Here's how the part is built. I have some questions about the finished solid (model axes, mm). Face numbers are marked on the shaded views. A direction names the side the tool comes from. Coordinates: 2 decimals unless noted, no trailing zeros. Loops run counter-clockwise (first coordinate to the right, second up) from the corner with the lowest first, then second, coordinate; pieces in that order, holes last. Notation, with made-up numbers: M -27.5,30.25 L -9.5,30.25 A24 cw -9.5,68.25 Z; hole C -6.5,38 d5. An arc over 180 degrees is marked long. Use one line per item in the form item = value. Start each with the question number.
(1) On a 3-axis mill with a long thin cutter (end or side, diameter ignored), from which of +Z, -Z, +X, -X, +Y, -Y can I reach the whole of each face in a straight line? I mean the marked faces 4, 5 and 6. Say none if no direction works.
(2) Imagine slicing it at C-C, the plane y = 38. Please give me the cut outline in (x, z), and give its area (3 significant figures).
(3) Thinking about a two-plate mould opening in Z: for the marked faces 1, 2 and 3, which applies, +Z half, -Z half, draft (parallel to the pull), parting line (faces both ways), or undercut?
(4) Imagine slicing it at B-B, the plane x = -43.5. Please give me the cut outline in (y, z).
(5) Imagine slicing it at D-D, the plane z = 31. Please give me the cut outline in (x, y).
(6) Please list where these lines run through material, in increasing order: L1, parallel to Z at x = 33, y = 51.5; L2, parallel to Z at x = 9, y = 14.5; L3, parallel to Y at x = -36.5, z = 63.5.
(7) Imagine slicing it at A-A, the plane y = 19. Please give me the cut outline in (x, z), and give its area (3 significant figures).
(8) Will these pins go through, and if not, where does the flat tip stop? P1, Ø4, axis at x = -13, z = 35.5, coming from the -Y side; P2, Ø9.5, axis at x = -26.5, z = 65.5, coming from the +Y side; P3, Ø1, axis at x = -31.5, y = 26.5, coming from the +Z side.
```python
from build123d import *

# Parameters (mm, degrees)
F0_W        = 100.3427430987
F0_H        = 68.4072636068
F1_DEPTH    = 75
F2_T1_DEPTH = 460.378361414
F3_W        = 100.3427430987
F3_H        = 24.6774237603
F4_DEPTH    = 25
F5_DEPTH    = 25


# Not quite as in the source:
# - a fillet or chamfer that OpenCascade refuses, or shapes differently, is made with other operations: its cross-section is extruded or revolved along the edge and cut away or added


with BuildPart() as f1:
    # F0 (on Top) → F1 (new body)
    with BuildSketch(Plane.XY):
        with Locations((-2.3588724434, -1.9959677011)):
            Rectangle(F0_W, F0_H)
    extrude(amount=F1_DEPTH)

    # F2: chamfer of 70 on 1 edges, made by hand

    # F2_s2 → F2_t1 (cut)
    with BuildSketch(Plane.YZ.offset(-232.5480531504)):
        Polygon((-36.1995995045, 5), (33.8004004955, 75), (-36.1995995045, 75), align=None)
    extrude(amount=F2_T1_DEPTH, mode=Mode.SUBTRACT)

    # F3 (on face) → F4 (cut)
    with BuildSketch(Plane(origin=(0, 32.2076641023, 0), x_dir=(-1, 0, 0), z_dir=(0, 1, 0))):
        with Locations((2.3588724434, 29.1229868308)):
            Rectangle(F3_W, F3_H)
    extrude(amount=-F4_DEPTH, mode=Mode.SUBTRACT)

    # F5 (add): a face of the model
    f5_faces = [f1.faces().sort_by_distance(p)[0] for p in [
        (-2.3588724434, 32.2076641023, 8.3921374753),
    ]]
    extrude(f5_faces, amount=F5_DEPTH)


solid = f1.part
```
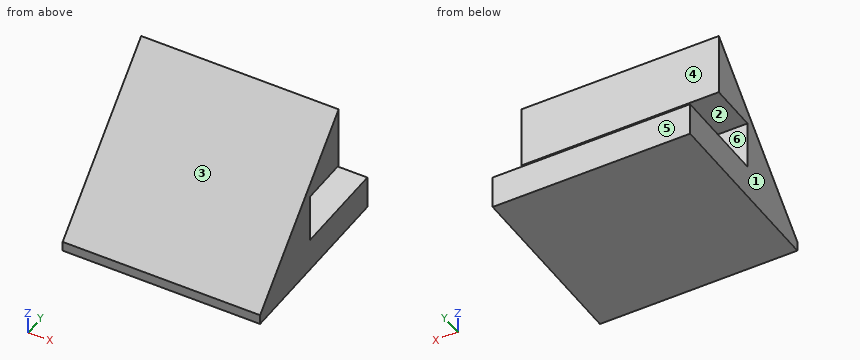
Answer:
q1.face_4 = +Z, +X, -X, +Y
q1.face_5 = +Z, -Z, +X, -X, +Y
q1.face_6 = +X, -X, +Y
q2.outline = M -52.53,0 L 47.81,0 L 47.81,16.78 L -52.53,16.78 Z
q2.area = 1,680 mm²
q3.face_1 = draft
q3.face_2 = undercut
q3.face_3 = +Z half
q4.outline = M -36.2,0 L 57.21,0 L 57.21,16.78 L 7.21,16.78 L 7.21,41.46 L 32.21,41.46 L 32.21,73.41 L -36.2,5 Z
q5.outline = M -52.53,-10.2 L 47.81,-10.2 L 47.81,7.21 L -52.53,7.21 Z
q6.L1 = 0 to 16.78
q6.L2 = 0 to 16.78, 41.46 to 55.7
q6.L3 = 22.3 to 32.21
q7.outline = M -52.53,0 L 47.81,0 L 47.81,16.78 L -52.53,16.78 Z; M -52.53,41.46 L 47.81,41.46 L 47.81,60.2 L -52.53,60.2 Z
q7.area = 3,560 mm²
q8.P1 = -7.7
q8.P2 = 32.21
q8.P3 = 68.2
